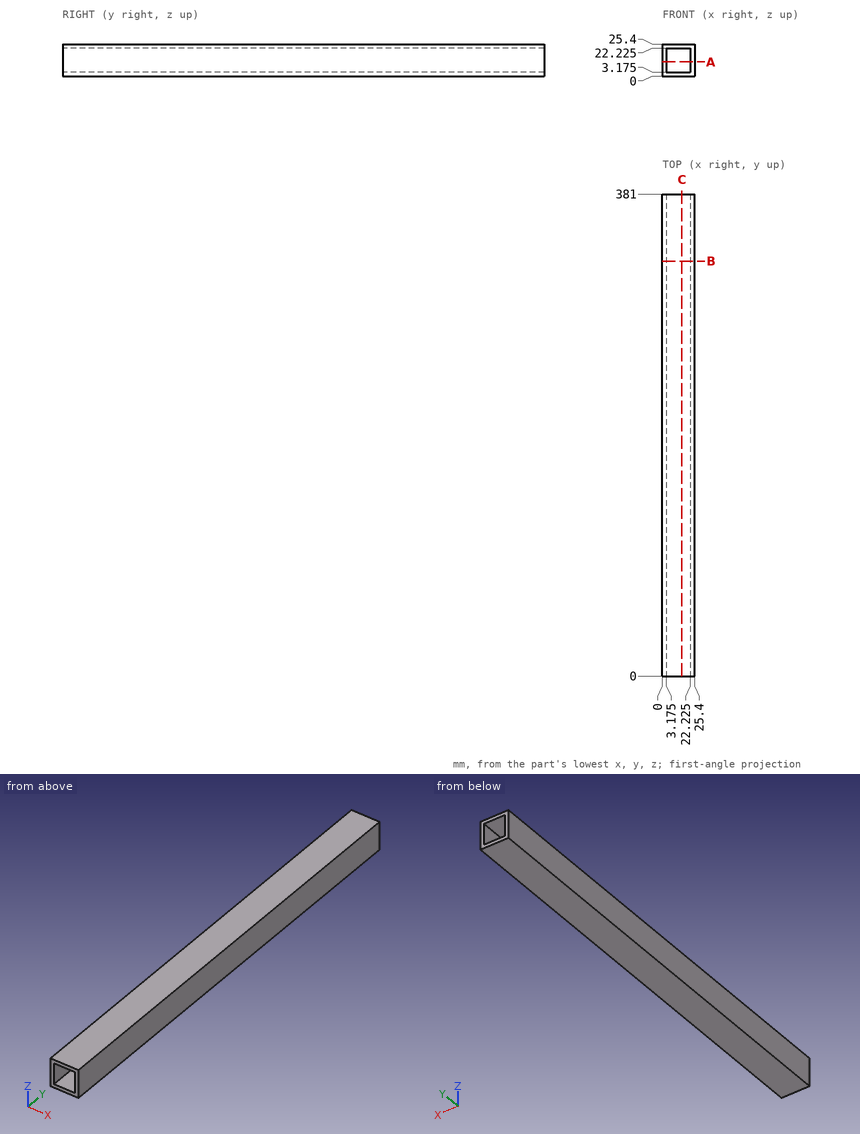
Print and shaded views of the part. All mm, measured from the part's lowest x, y and z. Coordinates: 2 decimals unless noted, no trailing zeros. Write each loop counter-clockwise with the first axis right and the second up, starting at its lowest first coordinate (ties: lowest second). Pieces come first, ordered by that corner, then holes.
(1) Cut at A-A, the plane z = 11.25. List the corners of the cut face in (x, y) (3 decimals).
(2) Drill centre line: probe 1 along Z at (x, y) = (3.75, 263.5) (3 decimals). Where is it in solid material? Low to high.
(3) Cut at C-C, the plane x = 15.5. List the corners of the cut face in (y, z) (3 decimals).
(4) Cut at B-B, the plane y = 328. List the corners of the cut face in (x, z) (3 decimals), and give its area (3 significant figures).
Geometry says:
1. outline: (0, 0) - (3.175, 0) - (3.175, 381) - (0, 381) - close; (22.225, 0) - (25.4, 0) - (25.4, 381) - (22.225, 381) - close
2. probe 1: z = 0 to 3.175, 22.225 to 25.4
3. outline: (0, 0) - (381, 0) - (381, 3.175) - (0, 3.175) - close; (0, 22.225) - (381, 22.225) - (381, 25.4) - (0, 25.4) - close
4. outline: (0, 0) - (25.4, 0) - (25.4, 25.4) - (0, 25.4) - close; hole (3.175, 3.175) - (22.225, 3.175) - (22.225, 22.225) - (3.175, 22.225) - close
4. area: 282 mm2
